```python
from build123d import *

# Parameters (mm, degrees)
F0_R     = 10
F1_DEPTH = 25


with BuildPart() as f1:
    # F0 (on Front) → F1 (new body, symmetric)
    with BuildSketch(Plane.XZ):
        with BuildLine():
            Line((-60, 0), (-90, 0))
            Line((-90, 0), (-90, -69.879413))
            ThreePointArc((-90, -69.879413), (-84.142136, -84.021549), (-70, -89.879413))
            Line((-70, -89.879413), (-60, -89.879413))
            Line((-60, -89.879413), (-60, -85.879413))
            ThreePointArc((-60, -85.879413), (-58.242641, -81.636772), (-54, -79.879413))
            Line((-54, -79.879413), (0, -79.879413))
            Line((0, -79.879413), (54, -79.879413))
            ThreePointArc((54, -79.879413), (58.242641, -81.636772), (60, -85.879413))
            Line((60, -85.879413), (60, -89.879413))
            Line((60, -89.879413), (70, -89.879413))
            ThreePointArc((70, -89.879413), (84.142136, -84.021549), (90, -69.879413))
            Line((90, -69.879413), (90, 0))
            Line((90, 0), (60, 0))
            ThreePointArc((60, 0), (42.426407, -42.426407), (0, -60))
            ThreePointArc((0, -60), (-42.426407, -42.426407), (-60, 0))
        make_face()
        with Locations((-70, -69.879413)):
            Circle(F0_R, mode=Mode.SUBTRACT)
        with Locations((70, -69.879413)):
            Circle(F0_R, mode=Mode.SUBTRACT)
    extrude(amount=F1_DEPTH, both=True)


solid = f1.part
```
The model under review builds one solid part; all positions refer to its coordinate system, in mm. A direction names the side the tool comes from. Round coordinates to 2 decimals unless told otherwise and drop trailing zeros. Write each loop counter-clockwise with the first axis right and the second up, starting at its lowest first coordinate (ties: lowest second). Pieces come first, ordered by that corner, then holes.
(1) We need section A-A on y = 19. Give the boundary of the cut face in (x, z).
(2) Insertion check: pin 1 (2 mm diameter, centred on x = 9.5, y = -13, fed in from +Z); pin 2 (8 mm diameter, centred on x = -30.5, y = -20, fed in from -Z); pin 3 (5 mm diameter, centred on x = 44.5, y = 18.5, fed in from +Z). Each pin has a flat end and moves straight along its axis. Give the tip position at first contact, or say it passes through.
(3) We need section D-D on z = -7. Give the boundary of the cut face in (x, y).
(4) Machinability: for faces 4 (the flat face through (-60, 0, -88)), 5 (the cylindrical face through (60.01, 0.35, -69.44)), which of the approach directions +Z, -Z, +X, -X, +Y, -Y give a long, thin tool a straight path to every point of the face, cutting with its end or side? Answer none if there is none.
(5) Mouldability with a two-part tool opening along Z and no side actions: class faces 1 (the flat face through (90, 0, -35)), 2 (the cylindrical face through (83.986, -0.35, -84.176)), 3 (the cylindrical face through (-79.99, 0.35, -69.44)) as +Z half, -Z half, draft (parallel to the pull), parting line (faces both ways), or undercut.
(6) Wall thickness on L1, parallel to X at y = -1.5, z = -69; L2, parallel to Z at x = 70, y = 0; L3, parallel to X at y = 22.5, z = -77: over which ranges is each line inside the solid? List them lowest first.
(7) We need section B-B on z = -30.5. Give the boundary of the cut face in (x, y), and give its area (3 significant figures).
(8) We need section C-C on x = 42.5. Give the boundary of the cut face in (y, z), and give its area (3 significant figures).
Findings below:
1. outline: (-90, -69.88) arc R20 ccw to (-70, -89.88) - (-60, -89.88) - (-60, -85.88) arc R6 cw to (-54, -79.88) - (54, -79.88) arc R6 cw to (60, -85.88) - (60, -89.88) - (70, -89.88) arc R20 ccw to (90, -69.88) - (90, 0) - (60, 0) arc R60 cw to (-60, 0) - (-90, 0) - close; hole circle Ø20 at (-70, -69.88); hole circle Ø20 at (70, -69.88)
2. pin 1: stops at z = -59.07
2. pin 2: stops at z = -79.88
2. pin 3: stops at z = -37.3
3. outline: (-90, -25) - (-59.59, -25) - (-59.59, 25) - (-90, 25) - close; (59.59, -25) - (90, -25) - (90, 25) - (59.59, 25) - close
4. face 4: -Z, +Y, -Y
4. face 5: +Y, -Y
5. face 1: draft
5. face 2: -Z half
5. face 3: undercut
6. L1: x = -90 to -79.96, -60.04 to 60.04, 79.96 to 90
6. L2: z = -89.88 to -79.88, -59.88 to 0
6. L3: x = -88.69 to -77.02, -62.98 to 62.98, 77.02 to 88.69
7. outline: (-90, -25) - (-51.67, -25) - (-51.67, 25) - (-90, 25) - close; (51.67, -25) - (90, -25) - (90, 25) - (51.67, 25) - close
7. area: 3,830 mm2
8. outline: (-25, -79.88) - (25, -79.88) - (25, -42.35) - (-25, -42.35) - close
8. area: 1,880 mm2
